Model file for the job. Use its own axes, mm. Face numbers are marked on the shaded views. A direction names the side the tool comes from. Coordinates: 2 decimals unless noted, no trailing zeros. Write each loop counter-clockwise with the first axis right and the second up, starting at its lowest first coordinate (ties: lowest second). Pieces come first, ordered by that corner, then holes. Notation, with made-up numbers: (12.5, 51) -> (62.5, 51) arc R4 ccw to (62.5, 57) -> close; hole circle Ø4 at (70, 64). An arc over 180 degrees is marked (long way). Answer as a JSON object with one key per item and string values. Group by question number.
from build123d import *

# Parameters (mm, degrees)
EXTRUDE1_DEPTH        = 25.4
EXTRUDE1_DEPTH_BACK   = 25.4
F_4_CLEARANCE_HOLE1_D = 3.4544
EXTRUDE2_DEPTH        = 49.26
LPATTERN1_COUNT       = 2
LPATTERN1_PITCH       = 25.4
FILLET2_R             = 9.525
CHAMFER1_SIZE         = 2.54


with BuildPart() as part:
    # Sketch1 → Extrude1 (new body, two sides)
    with BuildSketch(Plane.XY) as extrude1_sk:
        Polygon((0, 0), (48.26, 0), (48.26, 62.23), (35.56, 62.23), (35.56, 21.59), (0, 21.59), align=None)
    extrude(amount=EXTRUDE1_DEPTH)
    extrude(extrude1_sk.sketch, amount=-EXTRUDE1_DEPTH_BACK)

    # 4 Clearance Hole1 (through all)
    with Locations(Plane(origin=(0, 21.59, 0), x_dir=(-1, 0, 0), z_dir=(0, 1, 0))):
        with Locations((-5.08, -3.81), (-5.08, 3.81)):
            Hole(F_4_CLEARANCE_HOLE1_D / 2)

    # Sketch4 → Extrude2 (cut, through all)
    with BuildSketch(Plane(origin=(48.26, 0, 0), x_dir=(0, 0, -1), z_dir=(1, 0, 0))):
        with BuildLine():
            Line((16.0782, 50.8), (16.0782, 43.18))
            ThreePointArc((16.0782, 43.18), (12.7, 39.8018), (9.3218, 43.18))
            Line((9.3218, 43.18), (9.3218, 50.8))
            ThreePointArc((9.3218, 50.8), (12.7, 54.1782), (16.0782, 50.8))
        make_face()
    extrude2 = extrude(amount=-EXTRUDE2_DEPTH, mode=Mode.SUBTRACT)

    # LPattern1: Extrude2 ×2
    with Locations(*[(0, 0, i * LPATTERN1_PITCH) for i in range(1, LPATTERN1_COUNT)]):
        add(extrude2, mode=Mode.SUBTRACT)

    # Fillet2
    fillet2_edges = [part.edges().sort_by_distance(p)[0] for p in [
        (35.56, 21.59, 0),
    ]]
    fillet(fillet2_edges, radius=FILLET2_R)

    # Chamfer1
    chamfer1_edges = [part.edges().sort_by_distance(p)[0] for p in [
        (48.26, 31.115, -25.4),
        (0, 10.795, 25.4),
        (48.26, 31.115, 25.4),
        (0, 10.795, -25.4),
    ]]
    chamfer(chamfer1_edges, length=CHAMFER1_SIZE)


solid = part.part
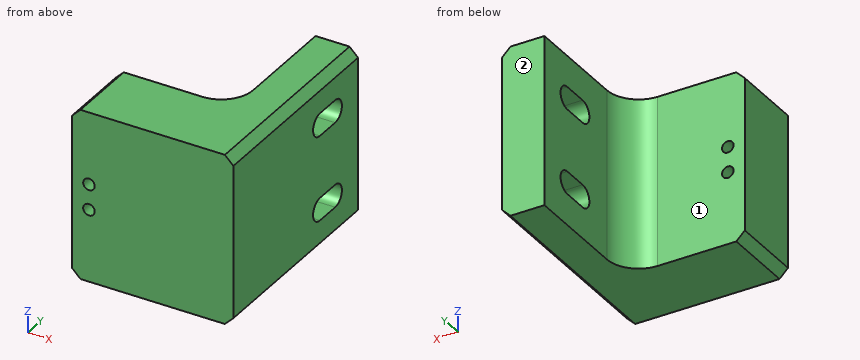
(1) 3-axis set-ups, long thin cutter, end or side, ignore diameter. For the marked faces 1 and 2: which of +Z, -Z, +X, -X, +Y, -Y reach the whole face in a straight line?
(2) Cut at B-B on x = 5.08. List the corners of the cut face in (y, z).
(3) Cut at D-D on z = 0.5. List the corners of the cut face in (x, y) (3 decimals), plus the area to 3 significant figures.
(4) Wall check: probe 1 along Z at (x, y) = (5, 12); probe 2 along Z at (x, y) = (4.5, 13); probe 3 along Y at (x, z) = (23, 3). Give the ranges that are in metal, low to high.
(5) Pin check, flat tips, straight feed: pin 1 (12 mm diameter, centred on x = 24.5, z = -18, fed in from -Y); pin 2 (10 mm diameter, centred on x = 22.5, z = -14.5, fed in from +Y); pin 3 (15.5 mm diameter, centred on y = 42, z = 7.5, fed in from -X); pin 4 (12 mm diameter, centred on x = 13, z = -9, fed in from +Y). Stop position of each tip, or through.
(6) Cut at C-C on x = 42. List the corners of the cut face in (y, z), plus the area to 3 significant figures.
(7) Cut at A-A on z = 12.7. List the corners of the cut face in (x, y) (3 decimals).
Results found:
{
 "1": {"face 1": "+Z, -Z, -X, +Y", "face 2": "+Z, -Z, +X, -X, +Y"},
 "2": {"outline": "(0, -25.4) -> (21.59, -25.4) -> (21.59, -5.54) -> (0, -5.54) -> close; (0, -2.08) -> (21.59, -2.08) -> (21.59, 2.08) -> (0, 2.08) -> close; (0, 5.54) -> (21.59, 5.54) -> (21.59, 25.4) -> (0, 25.4) -> close"},
 "3": {"outline": "(0, 0) -> (48.26, 0) -> (48.26, 62.23) -> (35.56, 62.23) -> (35.56, 31.115) arc R9.525 cw to (26.035, 21.59) -> (0, 21.59) -> close", "area": "1,580 mm²"},
 "4": {"probe 1": "z = -25.4 to -5.54, -2.08 to 2.08, 5.54 to 25.4", "probe 2": "z = -25.4 to -5.44, -2.18 to 2.18, 5.44 to 25.4", "probe 3": "y = 0 to 21.59"},
 "5": {"pin 1": "stops at y = 0", "pin 2": "stops at y = 21.7", "pin 3": "stops at x = 35.56", "pin 4": "stops at y = 21.59"},
 "6": {"outline": "(0, -25.4) -> (62.23, -25.4) -> (62.23, 25.4) -> (0, 25.4) -> close; hole (43.18, -16.08) -> (50.8, -16.08) arc R3.38 ccw to (50.8, -9.32) -> (43.18, -9.32) arc R3.38 ccw to start; hole (43.18, 9.32) -> (50.8, 9.32) arc R3.38 ccw to (50.8, 16.08) -> (43.18, 16.08) arc R3.38 ccw to start", "area": "2,990 mm²"},
 "7": {"outline": "(0, 0) -> (48.26, 0) -> (48.26, 39.802) -> (35.56, 39.802) -> (35.56, 31.115) arc R9.525 cw to (26.035, 21.59) -> (0, 21.59) -> close; (35.56, 54.178) -> (48.26, 54.178) -> (48.26, 62.23) -> (35.56, 62.23) -> close"}
}
